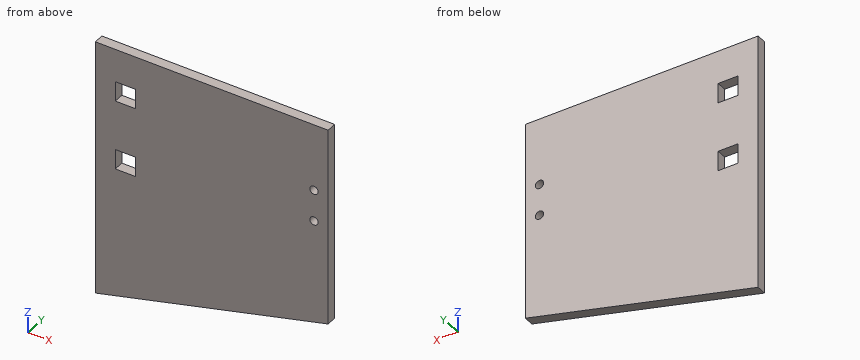
Autodesk Inventor part; units mm, degrees
ref_plane "YZ Plane" through (0, 0, 0) normal (1, 0, 0) x (0, 1, 0)
ref_plane "XZ Plane" through (0, 0, 0) normal (0, 1, 0) x (-1, 0, 0)
ref_plane "XY Plane" through (0, 0, 0) normal (0, 0, 1) x (1, 0, 0)
sketch "Sketch1" plane through (0, 0, 0) normal (0, 1, 0) x (-1, 0, 0)
  line L0 (0, 0) -> (-70, 0)
  line L1 (-70, 0) -> (-70, -60)
  line L2 (-70, -60) -> (0, -60)
  line L3 (0, -60) -> (0, 0)
  line L4 (0, -60) -> (0, -77.7966)
  line L5 (0, -77.7966) -> (-70, -60)
  dimension "d0" = 70
  dimension "d1" = 60
  dimension "d23" = 14.264
extrude "Extrusion1" add sketch "Sketch1" along normal blind 3
sketch "Sketch3" plane through (0, 3, 0) normal (0, 1, 0) x (1, 0, 0)
  circle A0 centre (65.75, 20.25) radius 1.25
  circle A1 centre (65.75, 29.75) radius 1.25
  line L0 (70, 0) -> (70, 60)
  line L1 (0, 0) -> (70, 0)
  line L2 (6, 10) -> (12, 10)
  line L3 (12, 10) -> (12, 16)
  line L4 (12, 16) -> (6, 16)
  line L5 (6, 16) -> (6, 10)
  line L6 (6, 37) -> (12, 37)
  line L7 (12, 37) -> (12, 31)
  line L8 (12, 31) -> (6, 31)
  line L9 (6, 31) -> (6, 37)
  line L10 (0, 77.7966) -> (0, 0)
  dimension "d15" = 2.5
  dimension "d16" = 4.25
  dimension "d17" = 4.25
  dimension "d18" = 2.5
  dimension "d19" = 20.25
  dimension "d20" = 9.5
  dimension "d24" = 6
  dimension "d25" = 6
  dimension "d26" = 6
  dimension "d27" = 10
  dimension "d28" = 15
  dimension "d29" = 6
extrude "Extrusion3" cut sketch "Sketch3" along normal through all both and the other way through all
equation "\"d17\" = d16"
equation "\"d18\" = d15"
properties part number "pinball-case-left-wall-outer-scaled"
Build history of the part. All positions in model axes, mm. Coordinates: 2 decimals unless noted, no trailing zeros. Write each loop counter-clockwise with the first axis right and the second up, starting at its lowest first coordinate (ties: lowest second). Pieces come first, ordered by that corner, then holes.
(1) Drill centre lines: line 1 (X direction, y = 2.05, z = -12.5); line 2 (X direction, y = 2, z = -20.25); line 3 (Z direction, x = 65.75, y = 1.15). Where is each one in solid material? Low to high.
(2) Cut at B-B on y = 0.55. List the corners of the cut face in (x, z).
(3) Cut at A-A on z = -20.25. List the corners of the cut face in (x, y).
(4) Pin check, flat tips, straight feed: pin 1 Ø1.5 at (x, y) = (8, 1) entering from -Z; pin 2 Ø2 at (x, z) = (65.75, -29.75) entering from +Y; pin 3 Ø0.9 at (x, y) = (8.5, 2) entering from -Z; pin 4 Ø1.5 at (x, y) = (10.5, 1.5) entering from -Z. Stop position of each tip, or through.
(5) Cut at D-D on z = -63. List the corners of the cut face in (x, y), and give its area (3 significant figures).
(6) Cut at C-C on x = 65.75. List the corners of the cut face in (y, z), and give its area (3 significant figures).
Working result:
1. line 1: x = 0 to 6, 12 to 70
1. line 2: x = 0 to 64.5, 67 to 70
1. line 3: z = -61.08 to -31, -28.5 to -21.5, -19 to 0
2. outline: (0, -77.8) - (70, -60) - (70, 0) - (0, 0) - close; hole (6, -37) - (12, -37) - (12, -31) - (6, -31) - close; hole (6, -16) - (12, -16) - (12, -10) - (6, -10) - close; hole circle Ø2.5 at (65.75, -29.75); hole circle Ø2.5 at (65.75, -20.25)
3. outline: (0, 0) - (64.5, 0) - (64.5, 3) - (0, 3) - close; (67, 0) - (70, 0) - (70, 3) - (67, 3) - close
4. pin 1: stops at z = -75.95
4. pin 2: passes through
4. pin 3: stops at z = -75.75
4. pin 4: stops at z = -75.32
5. outline: (0, 0) - (58.2, 0) - (58.2, 3) - (0, 3) - close
5. area: 175 mm2
6. outline: (0, -61.08) - (3, -61.08) - (3, -31) - (0, -31) - close; (0, -28.5) - (3, -28.5) - (3, -21.5) - (0, -21.5) - close; (0, -19) - (3, -19) - (3, 0) - (0, 0) - close
6. area: 168 mm2
